```python
from build123d import *

# Parameters (mm, degrees)
SKETCH_1_W               = 36
SKETCH_1_H               = 36
BODY_DEPTH               = 1.6
SKETCH_2_R               = 1.65
BOLTHOLE_M3_PILLAR_DEPTH = 26.506077707
FILLET_1_R               = 2
SKETCH_4_W               = 15
SKETCH_4_H               = 5.5
SKETCH_4_W_2             = 25
SKETCH_4_H_2             = 3
CONNECTORS_POWER_DEPTH   = 1.6
FILLET_3_R               = 1


with BuildPart() as part:
    # 스케치1 → Body (new body)
    with BuildSketch(Plane.XY):
        Rectangle(SKETCH_1_W, SKETCH_1_H)
    extrude(amount=BODY_DEPTH)

    # 스케치2 → BoltHole_M3_pillar (cut, through all)
    with BuildSketch(Plane.XY.offset(1.6)):
        with Locations((-15, 15)):
            Circle(SKETCH_2_R)
        with Locations((15, 15)):
            Circle(SKETCH_2_R)
        with Locations((15, -15)):
            Circle(SKETCH_2_R)
        with Locations((-15, -15)):
            Circle(SKETCH_2_R)
    extrude(amount=-BOLTHOLE_M3_PILLAR_DEPTH, mode=Mode.SUBTRACT)

    # 필렛1
    fillet_1_edges = [part.edges().sort_by_distance(p)[0] for p in [
        (-18, 18, 0.8),
        (18, 18, 0.8),
        (18, -18, 0.8),
        (-18, -18, 0.8),
    ]]
    fillet(fillet_1_edges, radius=FILLET_1_R)

    # 스케치4 → Connectors_power (add)
    with BuildSketch(Plane.XY):
        Polygon((-18, 12.5), (-25, 12.5), (-25, -4.5), (-22, -4.5), (-22, -12.5), (-18, -12.5), (-18, -4.5), align=None)
        Polygon((25, 12.5), (25, -4.5), (22, -4.5), (22, -12.5), (18, -12.5), (18, -4.5), (18, 12.5), align=None)
        with Locations((0, 20.75)):
            Rectangle(SKETCH_4_W, SKETCH_4_H)
        with Locations((0, -19.5)):
            Rectangle(SKETCH_4_W_2, SKETCH_4_H_2)
    extrude(amount=CONNECTORS_POWER_DEPTH)

    # 필렛3
    fillet_3_edges = [part.edges().sort_by_distance(p)[0] for p in [
        (12.5, -18, 0.8),
        (12.5, -21, 0.8),
        (-12.5, -21, 0.8),
        (-12.5, -18, 0.8),
        (-18, -12.5, 0.8),
        (-22, -12.5, 0.8),
        (-22, -4.5, 0.8),
        (-25, -4.5, 0.8),
        (-25, 12.5, 0.8),
        (-18, 12.5, 0.8),
        (25, -4.5, 0.8),
        (22, -4.5, 0.8),
        (22, -12.5, 0.8),
        (18, -12.5, 0.8),
        (18, 12.5, 0.8),
        (25, 12.5, 0.8),
        (7.5, 23.5, 0.8),
        (7.5, 18, 0.8),
        (-7.5, 18, 0.8),
        (-7.5, 23.5, 0.8),
    ]]
    fillet(fillet_3_edges, radius=FILLET_3_R)


solid = part.part
```
Geometry check sheet. Reference: the model listing, model coordinates, mm. A direction names the side the tool comes from. Give positions to 0.01 mm unless a question says otherwise; leave off trailing zeros. Loops run counter-clockwise (first coordinate to the right, second up) from the corner with the lowest first, then second, coordinate; pieces in that order, holes last. Notation, with made-up numbers: M -3,32.25 L 3,32.25 A26 cw 3,48.25 Z; hole C -38,29.25 d10. An arc over 180 degrees is marked long. Answer as CSV lines item,"result".
Item 1: Release check for a two-part mould opening along Y. For faces 1 (the flat face through (15, -18, 1)), 2 (the cylindrical face through (-17.43, 17.4, 0.81)), 3 (the cylindrical face through (16.574, -14.504, 0.811)) record: pulls with the +Y half, pulls with the -Y half, needs draft (parallel to the pull), parting line crosses it, or undercut.
Values:
face 1,"pulls with the -Y half"
face 2,"pulls with the +Y half"
face 3,"undercut"
Item 2: Cross-section at A-A on x = -15. Record the cut outline in (y, z), and give its area (3 significant figures).
Values:
outline,"M -18,0 L -16.65,0 L -16.65,1.6 L -18,1.6 Z; M -13.35,0 L 13.35,0 L 13.35,1.6 L -13.35,1.6 Z; M 16.65,0 L 18,0 L 18,1.6 L 16.65,1.6 Z"
area,"47.0 mm²"
Item 3: Depth check by flat-ended pin: P1, Ø0.8, axis at x = -23.5, z = 1, coming from the -Y side; P2, Ø0.8, axis at y = 20.5, z = 1, coming from the -X side; P3, Ø0.5, axis at y = -15.5, z = 1, coming from the -X side. Enter the tip coordinate at first touch or a pass-through.
Values:
P1,"stops at y = -4.5"
P2,"stops at x = -7.5"
P3,"stops at x = -18"
Item 4: Material ranges on line 1 (Y direction, x = -15, z = 0.55); line 2 (Y direction, x = -13.5, z = 0.7); line 3 (X direction, y = -7, z = 1.45), recorded low to high.
Values:
line 1,"y = -18 to -16.65, -13.35 to 13.35, 16.65 to 18"
line 2,"y = -18 to -15.69, -14.31 to 14.31, 15.69 to 18"
line 3,"x = -22 to 22"
Item 5: Cross-section at C-C on z = 0.5. Count the separate pieces of the cut face and the enclosed holes in it, and give its area (3 significant figures).
Values:
separate pieces,"1"
enclosed holes,"4"
area,"1,720 mm²"
Item 6: Access from +Z, -Z, +X, -X, +Y, -Y to the whole of each face (thin tool, end or side, straight path). Record for faces 4 (the flat face through (18, -15, 1)), 5 (the flat face through (18, 15, 1)), 6 (the flat face through (-18, -15, 1)), 7 (the flat face through (-18, 15, 1)), 8 (the flat face through (0, -21, 1)).
Values:
face 4,"+Z, -Z, +X, -Y"
face 5,"+Z, -Z, +X, +Y"
face 6,"+Z, -Z, -X, -Y"
face 7,"+Z, -Z, -X, +Y"
face 8,"+Z, -Z, +X, -X, -Y"
